Geometry: final body of the model. Coordinates: model frame, mm. Face numbers are marked on the shaded views. A direction names the side the tool comes from. Coordinates: 2 decimals unless noted, no trailing zeros. Order: outer loops, then holes, each group sorted by start corner. A loop starts at its lowest first (then second) coordinate and runs counter-clockwise, first axis right, second up. Notation, with made-up numbers: M 18,-37 L 47,-37 A22 cw 47,0 Z; hole C -33.75,-26 d5. An arc over 180 degrees is marked long. Write item = value, one per line.
from build123d import *

# Parameters (mm, degrees)
PAD_DEPTH       = 36
SKETCH001_W     = 41.77589
SKETCH001_H     = 44.999783
POCKET_DEPTH    = 10.5
SKETCH002_R     = 2.75
POCKET001_DEPTH = 36.001
FILLET_R        = 4
FILLET001_R     = 2
SKETCH003_R     = 2.85
HOLE_DEPTH      = 16.001
FILLET002_R     = 6
CHAMFER_SIZE    = 2
POCKET002_DEPTH = 3


with BuildPart() as part:
    # Sketch → Pad (new body)
    with BuildSketch(Plane.XZ):
        with BuildLine():
            Line((-20, 0), (20, 0))
            Line((20, 10), (20, 0))
            Line((10, 10), (20, 10))
            Line((10, 30), (10, 10))
            ThreePointArc((10, 30), (0, 40), (-10, 30))
            Line((-10, 10), (-10, 30))
            Line((-20, 10), (-10, 10))
            Line((-20, 0), (-20, 10))
        make_face()
    extrude(amount=PAD_DEPTH)

    # Sketch001 (on DatumPlane) → Pocket (cut, symmetric)
    with BuildSketch(Plane(origin=(0, -18, 0), x_dir=(1, 0, 0), z_dir=(0, 1, 0))):
        with Locations((0.131337, -40.390176)):
            Rectangle(SKETCH001_W, SKETCH001_H)
    extrude(amount=POCKET_DEPTH, both=True, mode=Mode.SUBTRACT)

    # Sketch002 (on Face4 of Pocket) → Pocket001 (cut, through all)
    with BuildSketch(Plane(origin=(0, 0, 0), x_dir=(1, 0, 0), z_dir=(0, 1, 0))):
        with Locations((0, -30)):
            Circle(SKETCH002_R)
    extrude(amount=-POCKET001_DEPTH, mode=Mode.SUBTRACT)

    # Fillet
    fillet_edges = [part.edges().sort_by_distance(p)[0] for p in [
        (10, -18, 17.890285),
        (-10, -18, 17.890285),
    ]]
    fillet(fillet_edges, radius=FILLET_R)

    # Fillet001
    fillet001_edges = [part.edges().sort_by_distance(p)[0] for p in [
        (10, -18, 10),
        (-10, -18, 10),
    ]]
    fillet(fillet001_edges, radius=FILLET001_R)

    # Sketch003 (on DatumPlane) → Hole (cut, through all)
    with BuildSketch(Plane(origin=(0, 0, 16), x_dir=(1, 0, 0), z_dir=(0, 0, -1))):
        with Locations((15, 18)):
            Circle(SKETCH003_R)
        with Locations((-15, 18)):
            Circle(SKETCH003_R)
    extrude(amount=HOLE_DEPTH, mode=Mode.SUBTRACT)

    # Fillet002
    fillet002_edges = [part.edges().sort_by_distance(p)[0] for p in [
        (20, 0, 5),
        (-20, 0, 5),
        (-20, -36, 5),
        (20, -36, 5),
    ]]
    fillet(fillet002_edges, radius=FILLET002_R)

    # Chamfer
    chamfer_edges = [part.edges().sort_by_distance(p)[0] for p in [
        (-2.75, 0, 30),
    ]]
    chamfer(chamfer_edges, length=CHAMFER_SIZE)

    # Sketch004 (on Face15 of Chamfer) → Pocket002 (cut)
    with BuildSketch(Plane.XZ.offset(36)):
        Polygon((-0.093793, 34.5), (-3.944011, 32.168773), (-3.850218, 27.668773), (0.093793, 25.5), (3.944011, 27.831227), (3.850218, 32.331227), align=None)
    extrude(amount=-POCKET002_DEPTH, mode=Mode.SUBTRACT)


solid = part.part
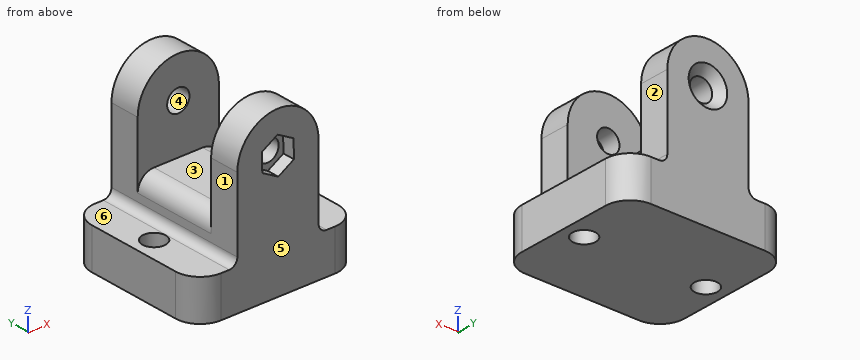
1) Pin query (flat end, axial travel): pin 1 (1.5 mm diameter, centred on x = -8, y = -20.5, fed in from +Z); pin 2 (1 mm diameter, centred on x = -1.5, z = 28, fed in from -Y); pin 3 (6.5 mm diameter, centred on x = 14.5, y = -24, fed in from +Z). Return the tip coordinate at first contact, or that it passes through.
Numbers:
pin_1 = 17.69
pin_2 = -33
pin_3 = 10.15
2) Set-up query: the marked faces 1, 2 and 3. Return all of +Z, -Z, +X, -X, +Y, -Y with unobstructed straight access to the full face (end or side cutting, diameter ignored); none if empty.
Numbers:
face_1 = +Z, -X, +Y, -Y
face_2 = +Z, +X, +Y, -Y
face_3 = +Z, +X, -X
3) Mould query, pull axis Z, two halves, no side actions, for the marked faces 4, 5 and 6. Classes: pulls with the +Z half, pulls with the -Z half, needs draft (parallel to the pull), parting line crosses it, or undercut.
Numbers:
face_4 = undercut
face_5 = needs draft
face_6 = pulls with the +Z half
4) Section A-A, the plane z = 22. Return loops of the section in (x, y).
Numbers:
outline = M -10,-36 L 10,-36 L 10,-28.5 L -10,-28.5 Z; M -10,-7.5 L 10,-7.5 L 10,0 L -10,0 Z
5) Section D-D, the plane z = 5. Return loops of the section in (x, y).
Numbers:
outline = M -20,-30 A6 ccw -14,-36 L 14,-36 A6 ccw 20,-30 L 20,-6 A6 ccw 14,0 L -14,0 A6 ccw -20,-6 Z; hole C -15,-18 d5.7; hole C 15,-18 d5.7
6) Section B-B, the plane y = -18. Return loops of the section in (x, z).
Numbers:
outline = M -20,0 L -17.85,0 L -17.85,10 L -20,10 Z; M -12.15,0 L 12.15,0 L 12.15,10 L 12,10 A2 cw 10,12 L 10,13.89 A4 ccw 6,17.89 L -6,17.89 A4 ccw -10,13.89 L -10,12 A2 cw -12,10 L -12.15,10 Z; M 17.85,0 L 20,0 L 20,10 L 17.85,10 Z
7) Section C-C, the plane x = -15. Return loops of the section in (y, z).
Numbers:
outline = M -35.92,0 L -20.85,0 L -20.85,10 L -35.92,10 Z; M -15.15,0 L -0.08,0 L -0.08,10 L -15.15,10 Z
8) Line query: L1, parallel to Y at x = 4.5, z = 27; L2, parallel to X at y = -5.3, z = 30; L3, parallel to Z at x = 0, y = -30. Output: solid intervals per line, ascending.
Numbers:
L1 = -36 to -28.5, -7.5 to 0
L2 = -10 to -2.75, 2.75 to 10
L3 = 0 to 27.25, 32.75 to 40
